from build123d import *

# Parameters (mm, degrees)
F0_W     = 38.1
F0_H     = 50.8
F1_DEPTH = 584.2
F2_W     = 38.1
F2_H     = 6.35
F3_DEPTH = 38.1


with BuildPart() as f1:
    # F0 (on Right) → F1 (new body)
    with BuildSketch(Plane.YZ):
        Rectangle(F0_W, F0_H)
    extrude(amount=F1_DEPTH)

    # F2 (on face) → F3 (cut, through all)
    with BuildSketch(Plane.XZ.offset(19.05)):
        with Locations((158.75, 22.225)):
            Rectangle(F2_W, F2_H)
        with Locations((425.45, 22.225)):
            Rectangle(F2_W, F2_H)
    extrude(amount=-F3_DEPTH, mode=Mode.SUBTRACT)


solid = f1.part
Model file for the job. Use its own axes, mm. A direction names the side the tool comes from. Give positions to 0.01 mm unless a question says otherwise; leave off trailing zeros. Order: outer loops, then holes, each group sorted by start corner. A loop starts at its lowest first (then second) coordinate and runs counter-clockwise, first axis right, second up. Notation, with made-up numbers: M -4.5,59.5 L 2.5,59.5 A20 cw 2.5,72.5 Z; hole C 53.25,2.25 d2. An arc over 180 degrees is marked long. Put each result on its own line as item: value. Start each with the question number.
(1) Pin check, flat tip, straight feed: pin 1 Ø19 at (x, y) = (166, 4) entering from +Z. Stop position of the tip, or through.
(2) Pull direction X, two halves, no side cores. Call faces 1 (the face through (425, 0, 19.05)), 2 (the face through (0, 0, 0)), 3 (the face through (290, 0, 25.4)): released by +X, released by -X, zero draft, split by the parting line, or undercut.
(3) Tool access for faces 4 (the face through (513, 0, 25.4)), 5 (the face through (158, 0, 19.05)): list every direction of +Z, -Z, +X, -X, +Y, -Y with a clear straight run to the whole face (end or side of a thin tool).
(4) Band-saw the part on A-A on y = 6. Give the cut face in (x, z).
(5) Drill centre lines: L1, parallel to X at y = -1, z = 22.5; L2, parallel to Z at x = 434, y = -6. Where is each one in solid material? Low to high. Write a range as [from, to].
Results below:
1. pin 1: stops at z = 19.05
2. face 1: undercut
2. face 2: released by -X
2. face 3: zero draft
3. face 4: +Z, +X, -X, +Y, -Y
3. face 5: +Z, +Y, -Y
4. outline: M 0,-25.4 L 584.2,-25.4 L 584.2,25.4 L 444.5,25.4 L 444.5,19.05 L 406.4,19.05 L 406.4,25.4 L 177.8,25.4 L 177.8,19.05 L 139.7,19.05 L 139.7,25.4 L 0,25.4 Z
5. L1: x = [0, 139.7], [177.8, 406.4], [444.5, 584.2]
5. L2: z = [-25.4, 19.05]
